The model under review builds one solid part; all positions refer to its coordinate system, in mm. A direction names the side the tool comes from. Coordinates: 2 decimals unless noted, no trailing zeros. Loops run counter-clockwise (first coordinate to the right, second up) from the corner with the lowest first, then second, coordinate; pieces in that order, holes last. Notation, with made-up numbers: (68, 85.25) - (88, 85.25) arc R10 cw to (88, 96.25) - close; hole circle Ø6 at (0.25, 46). An arc over 180 degrees is marked (long way). Use a Markdown table: item, result. Add a question column.
1) The part is to be moulded in two halves that separate along Y. For faces 4 (the flat face through (-94, -1, -7)), 5 (the cylindrical face through (-86.16, 56.05, -4.44)), 6 (the cylindrical face through (-92.57, -58, -7.6)), say which applies: pulls with the +Y half, pulls with the -Y half, needs draft (parallel to the pull), parting line crosses it, or undercut.
2) Add section D-D, the plane z = -2. Give the boundary of the cut face in (x, y).
3) Clearance check with flat-ended pins moving along their axes: pin 1 (3.5 mm diameter, centred on x = 89.5, y = -55, fed in from -Z); pin 2 (5.5 mm diameter, centred on x = -88.5, y = -53.5, fed in from +Z); pin 3 (2 mm diameter, centred on x = 90.5, y = -53.5, fed in from +Z). State where each tip first meets the part, or that it passes through.
4) Add section B-B, the plane x = -38. Give the boundary of the cut face in (y, z).
5) For faces 1 (the flat face through (-1, -59.5, -7)), 2 (the flat face through (-88, -57, -9)), 3 (the cylindrical face through (-72.5, -38.07, -7.6)), list the 3-axis set-ups (+Z, -Z, +X, -X, +Y, -Y) from which the entire face can be reached by the end or side of a thin tool; tool diameter is ignored.
6) To check wall thickness, follow L1, parallel to Y at x = 89.5, z = -12.55; L2, parallel to Y at x = -89.5, z = -6.5; L3, parallel to Y at x = -2.5, z = -9. State the ranges of each line that lie inside material, in increasing order. Write a range as [from, to].
7) Add section A-A, the plane y = -17.5. Give the boundary of the cut face in (x, z), and give its area (3 significant figures).
8) Add section C-C, the plane z = -13. Give the boundary of the cut face in (x, y).
```python
from build123d import *

# Parameters (mm, degrees)
F0_W     = 188
F0_H     = 119
F0_R     = 3.5
F0_W_2   = 148
F0_H_2   = 79
F0_R_2   = 2
F1_DEPTH = 15
F2_DEPTH = 9
F3_R     = 5


with BuildPart() as f1:
    # F0 (on Top) → F1 (new body)
    with BuildSketch(Plane.XY):
        Rectangle(F0_W, F0_H)
        with Locations((-89.5, -55)):
            Circle(F0_R, mode=Mode.SUBTRACT)
        with Locations((89.5, -55)):
            Circle(F0_R, mode=Mode.SUBTRACT)
        with Locations((-89.5, 55)):
            Circle(F0_R, mode=Mode.SUBTRACT)
        Rectangle(F0_W_2, F0_H_2, mode=Mode.SUBTRACT)
        with Locations((89.5, 55)):
            Circle(F0_R, mode=Mode.SUBTRACT)
        with Locations((-89.5, 55)):
            Circle(F0_R)
        with Locations((-89.5, 55)):
            Circle(F0_R_2, mode=Mode.SUBTRACT)
        with Locations((89.5, 55)):
            Circle(F0_R)
        with Locations((89.5, 55)):
            Circle(F0_R_2, mode=Mode.SUBTRACT)
        with Locations((89.5, -55)):
            Circle(F0_R)
        with Locations((89.5, -55)):
            Circle(F0_R_2, mode=Mode.SUBTRACT)
        with Locations((-89.5, -55)):
            Circle(F0_R)
        with Locations((-89.5, -55)):
            Circle(F0_R_2, mode=Mode.SUBTRACT)
    extrude(amount=-F1_DEPTH)

    # F0 (on Top) → F2 (cut)
    with BuildSketch(Plane.XY):
        with Locations((-89.5, 55)):
            Circle(F0_R)
        with Locations((-89.5, 55)):
            Circle(F0_R_2, mode=Mode.SUBTRACT)
        with Locations((89.5, 55)):
            Circle(F0_R)
        with Locations((89.5, 55)):
            Circle(F0_R_2, mode=Mode.SUBTRACT)
        with Locations((89.5, -55)):
            Circle(F0_R)
        with Locations((89.5, -55)):
            Circle(F0_R_2, mode=Mode.SUBTRACT)
        with Locations((-89.5, -55)):
            Circle(F0_R)
        with Locations((-89.5, -55)):
            Circle(F0_R_2, mode=Mode.SUBTRACT)
    extrude(amount=-F2_DEPTH, mode=Mode.SUBTRACT)

    # F3
    f3_edges = [f1.edges().sort_by_distance(p)[0] for p in [
        (94, 59.5, -7.5),
        (-94, 59.5, -7.5),
        (-94, -59.5, -7.5),
        (94, -59.5, -7.5),
        (-74, 39.5, -7.5),
        (74, 39.5, -7.5),
        (74, -39.5, -7.5),
        (-74, -39.5, -7.5),
    ]]
    fillet(f3_edges, radius=F3_R)


solid = f1.part
```
From the geometry:
| question | item | result |
|---|---|---|
| 1 | face 4 | needs draft |
| 1 | face 5 | undercut |
| 1 | face 6 | pulls with the -Y half |
| 2 | outline | (-94, -54.5) arc R5 ccw to (-89, -59.5) - (89, -59.5) arc R5 ccw to (94, -54.5) - (94, 54.5) arc R5 ccw to (89, 59.5) - (-89, 59.5) arc R5 ccw to (-94, 54.5) - close; hole circle Ø7 at (-89.5, -55); hole circle Ø7 at (-89.5, 55); hole (-74, -34.5) arc R5 ccw to (-69, -39.5) - (69, -39.5) arc R5 ccw to (74, -34.5) - (74, 34.5) arc R5 ccw to (69, 39.5) - (-69, 39.5) arc R5 ccw to (-74, 34.5) - close; hole circle Ø7 at (89.5, -55); hole circle Ø7 at (89.5, 55) |
| 3 | pin 1 | passes through |
| 3 | pin 2 | stops at z = 0 |
| 3 | pin 3 | stops at z = -9 |
| 4 | outline | (-59.5, -15) - (-39.5, -15) - (-39.5, 0) - (-59.5, 0) - close; (39.5, -15) - (59.5, -15) - (59.5, 0) - (39.5, 0) - close |
| 5 | face 1 | +Z, -Z, +X, -X, -Y |
| 5 | face 2 | +Z |
| 5 | face 3 | +Z, -Z |
| 6 | L1 | y = [-59.47, -57], [-53, 53], [57, 59.47] |
| 6 | L2 | y = [-59.47, -58.5], [-51.5, 51.5], [58.5, 59.47] |
| 6 | L3 | y = [-59.5, -39.5], [39.5, 59.5] |
| 7 | outline | (-94, -15) - (-74, -15) - (-74, 0) - (-94, 0) - close; (74, -15) - (94, -15) - (94, 0) - (74, 0) - close |
| 7 | area | 600 mm^2 |
| 8 | outline | (-94, -54.5) arc R5 ccw to (-89, -59.5) - (89, -59.5) arc R5 ccw to (94, -54.5) - (94, 54.5) arc R5 ccw to (89, 59.5) - (-89, 59.5) arc R5 ccw to (-94, 54.5) - close; hole circle Ø4 at (-89.5, -55); hole circle Ø4 at (-89.5, 55); hole (-74, -34.5) arc R5 ccw to (-69, -39.5) - (69, -39.5) arc R5 ccw to (74, -34.5) - (74, 34.5) arc R5 ccw to (69, 39.5) - (-69, 39.5) arc R5 ccw to (-74, 34.5) - close; hole circle Ø4 at (89.5, -55); hole circle Ø4 at (89.5, 55) |
